Design review of the part built by this model. Coordinates are the model's own, in mm. Face numbers are marked on the shaded views. A direction names the side the tool comes from. Coordinates: 2 decimals unless noted, no trailing zeros. Loops run counter-clockwise (first coordinate to the right, second up) from the corner with the lowest first, then second, coordinate; pieces in that order, holes last. Notation, with made-up numbers: M -7.5,-4.5 L 51.5,-4.5 A21 ccw 51.5,21.5 Z; hole C 22,79.25 d6. An arc over 180 degrees is marked long. Answer as a JSON object with one key per item and string values. Group by question number.
1. Draft analysis for pull direction Y (two halves, no side actions). For the marked faces 1, 2 and 3, state which applies: +Y half, -Y half, draft (parallel to the pull), parting line (faces both ways), or undercut.
2. Insertion check: pin 1 (6.5 mm diameter, centred on x = 48, y = 48, fed in from +Z); pin 2 (3.5 mm diameter, centred on x = 1.5, y = -42.5, fed in from +Z). Each pin has a flat end and moves straight along its axis. Give the tip position at first contact, or say it passes through.
3. Machinability: for the marked faces 4, 5 and 6, which of the approach directions +Z, -Z, +X, -X, +Y, -Y give a long, thin tool a straight path to every point of the face, cutting with its end or side? Answer none if there is none.
4. Consider section C-C (x = 31.5). State the section outline as (y, z) points.
5. To check wall thickness, follow probe 1 along Y at (x, z) = (-48, 5.5); probe 2 along Y at (x, z) = (-33, -7.75); probe 3 along Y at (x, z) = (-5.5, 6.5). State the ranges of each line that lie inside material, in increasing order.
6. Consider section D-D (z = 7.5). Count the separate pieces of the cut face and the enclosed holes in it, then the cut area to 3 significant figures.
7. Consider section B-B (y = 26). State the section outline as (x, z) points, then the cut area to 3 significant figures.
8. Consider section A-A (x = 0). State the section outline as (y, z) points.
from build123d import *

# Parameters (mm, degrees)
SKETCH1_W           = 115
SKETCH1_H           = 115
BOSS_EXTRUDE1_DEPTH = 12.5
SKETCH2_R           = 4
CUT_EXTRUDE1_DEPTH  = 30
FILLET1_R           = 10
SKETCH5_W           = 88
SKETCH5_H           = 88
CUT_EXTRUDE3_DEPTH  = 30
FILLET4_R           = 10
SKETCH6_W           = 88
SKETCH6_H           = 20
BOSS_EXTRUDE2_DEPTH = 25
SKETCH14_W          = 22
SKETCH14_H          = 15
BOSS_EXTRUDE6_DEPTH = 30
SKETCH16_R          = 15.5
CUT_EXTRUDE7_DEPTH  = 30
FILLET6_R           = 1
FILLET8_R           = 2
SKETCH17_R          = 2.25
CUT_EXTRUDE8_DEPTH  = 40
SKETCH18_W          = 12
SKETCH18_H          = 12
CUT_EXTRUDE9_DEPTH  = 25


with BuildPart() as part:
    # Sketch1 → Boss-Extrude1 (new, symmetric)
    with BuildSketch(Plane.XY):
        Rectangle(SKETCH1_W, SKETCH1_H)
    extrude(amount=BOSS_EXTRUDE1_DEPTH, both=True)

    # Sketch2 → Cut-Extrude1 (cut)
    with BuildSketch(Plane.XY.offset(12.5)):
        with Locations((-48, 48)):
            Circle(SKETCH2_R)
        with Locations((48, 48)):
            Circle(SKETCH2_R)
        with Locations((48, -48)):
            Circle(SKETCH2_R)
        with Locations((-48, -48)):
            Circle(SKETCH2_R)
    extrude(amount=-CUT_EXTRUDE1_DEPTH, mode=Mode.SUBTRACT)

    # Fillet1
    fillet1_edges = [part.edges().sort_by_distance(p)[0] for p in [
        (-57.5, 57.5, 0),
        (57.5, 57.5, 0),
        (57.5, -57.5, 0),
        (-57.5, -57.5, 0),
    ]]
    fillet(fillet1_edges, radius=FILLET1_R)

    # Sketch5 → Cut-Extrude3 (cut)
    with BuildSketch(Plane.XY.offset(12.5)):
        Rectangle(SKETCH5_W, SKETCH5_H)
    extrude(amount=-CUT_EXTRUDE3_DEPTH, mode=Mode.SUBTRACT)

    # Fillet4
    fillet4_edges = [part.edges().sort_by_distance(p)[0] for p in [
        (-44, -44, 0),
        (-44, 44, 0),
        (44, 44, 0),
        (44, -44, 0),
    ]]
    fillet(fillet4_edges, radius=FILLET4_R)

    # Sketch6 → Boss-Extrude2 (add)
    with BuildSketch(Plane.XY.offset(12.5)):
        Rectangle(SKETCH6_W, SKETCH6_H)
    extrude(amount=-BOSS_EXTRUDE2_DEPTH)

    # Sketch14 → Boss-Extrude6 (add)
    with BuildSketch(Plane(origin=(0, -22.1, 0), x_dir=(-1, 0, 0), z_dir=(0, -1, 0))):
        with Locations((0, -5)):
            Rectangle(SKETCH14_W, SKETCH14_H)
    extrude(amount=BOSS_EXTRUDE6_DEPTH)

    # Sketch16 → Cut-Extrude7 (cut)
    with BuildSketch(Plane.XY.offset(12.5)):
        Circle(SKETCH16_R)
    extrude(amount=-CUT_EXTRUDE7_DEPTH, mode=Mode.SUBTRACT)

    # Fillet6
    fillet6_edges = [part.edges().sort_by_distance(p)[0] for p in [
        (-11.842719282, -10, 0),
        (11.842719282, -10, 0),
        (11.842719282, 10, 0),
        (-11.842719282, 10, 0),
    ]]
    fillet(fillet6_edges, radius=FILLET6_R)

    # Fillet8
    fillet8_edges = [part.edges().sort_by_distance(p)[0] for p in [
        (-44, -10, 0),
        (-44, 10, 0),
        (44, 10, 0),
        (44, -10, 0),
        (-11, -44, 5),
        (11, -44, 5),
        (11, -22.1, 5),
        (-11, -22.1, 5),
    ]]
    fillet(fillet8_edges, radius=FILLET8_R)

    # Sketch17 → Cut-Extrude8 (cut)
    with BuildSketch(Plane(origin=(0, -22.1, 0), x_dir=(1, 0, 0), z_dir=(0, 1, 0))):
        with Locations(Location((0, -7.5, 0), (0, 0, 180))):
            Circle(SKETCH17_R)
    extrude(amount=-CUT_EXTRUDE8_DEPTH, mode=Mode.SUBTRACT)

    # Sketch18 → Cut-Extrude9 (cut)
    with BuildSketch(Plane(origin=(0, -57.5, 0), x_dir=(-1, 0, 0), z_dir=(0, -1, 0))):
        with Locations((0, -7.5)):
            Rectangle(SKETCH18_W, SKETCH18_H)
    extrude(amount=-CUT_EXTRUDE9_DEPTH, mode=Mode.SUBTRACT)


solid = part.part
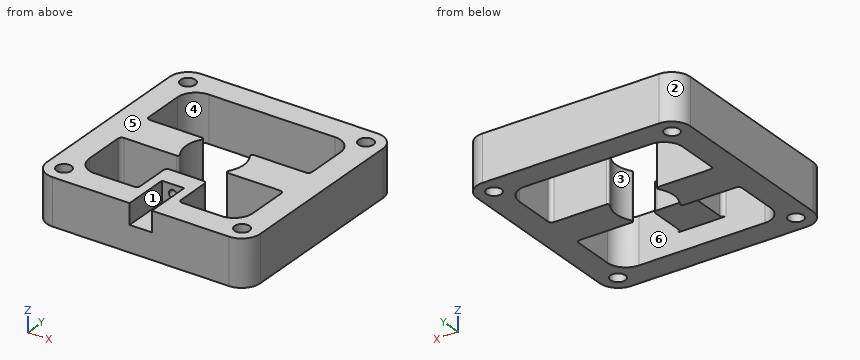
Findings below:
{
 "1": {"face 1": "draft", "face 2": "+Y half", "face 3": "undercut"},
 "2": {"pin 1": "passes through", "pin 2": "stops at z = 1.5"},
 "3": {"face 4": "+Z, -Z", "face 5": "+Z, +X, -X, +Y, -Y", "face 6": "-Z"},
 "4": {"outline": "M -57.5,-12.5 L -44,-12.5 L -44,12.5 L -57.5,12.5 Z; M -10,-12.5 L 10,-12.5 L 10,12.5 L -10,12.5 Z; M 44,-12.5 L 57.5,-12.5 L 57.5,12.5 L 44,12.5 Z"},
 "5": {"probe 1": "y = -57.49 to -52, -44 to 44, 52 to 57.49", "probe 2": "y = -57.5 to -44, -10 to 10, 44 to 57.5", "probe 3": "y = -32.5 to -22.1, 44 to 57.5"},
 "6": {"separate pieces": "1", "enclosed holes": "4", "area": "6,600 mm^2"},
 "7": {"outline": "M -57.5,-12.5 L -44,-12.5 L -44,12.5 L -57.5,12.5 Z; M 44,-12.5 L 57.5,-12.5 L 57.5,12.5 L 44,12.5 Z", "area": "675 mm^2"},
 "8": {"outline": "M -57.5,-12.5 L -44,-12.5 L -44,-2.5 L -22.1,-2.5 L -22.1,5.25 L -32.5,5.25 L -32.5,1.5 L -57.5,1.5 Z; M -32.5,9.75 L -22.1,9.75 L -22.1,12.5 L -32.5,12.5 Z; M 44,-12.5 L 57.5,-12.5 L 57.5,12.5 L 44,12.5 Z"}
}
